from build123d import *

# Parameters (mm, degrees)
BOSS_EXTRUDE1_DEPTH  = 66.675
M6_CLEARANCE_HOLE3_D = 6.6
LPATTERN1_COUNT      = 3
LPATTERN1_PITCH      = 44.45
FILLET1_R            = 2.54


with BuildPart() as part:
    # Sketch1 → Boss-Extrude1 (new, symmetric)
    with BuildSketch(Plane.XY):
        with BuildLine():
            Line((0, 0), (0, 25.4))
            Line((0, 25.4), (3.175, 25.4))
            Line((3.175, 25.4), (3.175, 4.445))
            ThreePointArc((3.175, 4.445), (3.546974388, 3.546974388), (4.445, 3.175))
            Line((4.445, 3.175), (25.4, 3.175))
            Line((25.4, 3.175), (25.4, 0))
            Line((25.4, 0), (0, 0))
        make_face()
    extrude(amount=BOSS_EXTRUDE1_DEPTH, both=True)

    # M6 Clearance Hole3 (through all)
    with Locations(Plane.XZ):
        with Locations((19.05, 60.325), (19.05, 44.45), (19.05, 28.575)):
            m6_clearance_hole3 = Hole(M6_CLEARANCE_HOLE3_D / 2)

    # LPattern1: M6 Clearance Hole3 ×3
    with Locations(*[(0, 0, -i * LPATTERN1_PITCH) for i in range(1, LPATTERN1_COUNT)]):
        add(m6_clearance_hole3, mode=Mode.SUBTRACT)

    # Fillet1
    fillet1_edges = [part.edges().sort_by_distance(p)[0] for p in [
        (1.5875, 25.4, 66.675),
        (1.5875, 25.4, -66.675),
        (25.4, 1.5875, 66.675),
        (25.4, 1.5875, -66.675),
    ]]
    fillet(fillet1_edges, radius=FILLET1_R)


solid = part.part
Part model, mm, in its own coordinate system. A direction names the side the tool comes from. Give positions to 0.01 mm unless a question says otherwise; leave off trailing zeros. Order: outer loops, then holes, each group sorted by start corner. A loop starts at its lowest first (then second) coordinate and runs counter-clockwise, first axis right, second up. Notation, with made-up numbers: (-4, -2) -> (55, -2) arc R26 cw to (55, 34) -> close; hole circle Ø8 at (17, 28). An arc over 180 degrees is marked (long way). Use one line per item in the form item = value.
(1) Saw through at D-D (y = 16.5). Write the cut outline in (x, z) (3 decimals), then the cut area to 3 significant figures.
Solution:
outline = (0, -66.675) -> (3.175, -66.675) -> (3.175, 66.675) -> (0, 66.675) -> close
area = 423 mm²
(2) Saw through at C-C (x = 19.05). Count the separate pieces of the cut face and the enclosed holes in it, then the cut area to 3 significant figures.
Solution:
separate_pieces = 10
enclosed_holes = 0
area = 235 mm²
(3) Flat gauge pins, fed straight in: P1, Ø10.5, axis at y = 18.5, z = -12.5, coming from the +X side (3 decimals); P2, Ø6.5, axis at x = 12.5, z = 13.5, coming from the +Y side (3 decimals); P3, Ø3, axis at x = 5.5, z = 17, coming from the +Y side. Where does each tip first touch, or does it go through?
Solution:
P1 = 3.175
P2 = 3.175
P3 = 3.26
(4) Tool access for faces 4 (the face through (10, 0, 1)), 5 (the face through (3.175, 15, 1)): list every direction of +Z, -Z, +X, -X, +Y, -Y with a clear straight run to the whole face (end or side of a thin tool).
Solution:
face_4 = +Z, -Z, +X, -X, -Y
face_5 = +Z, -Z, +X, +Y
(5) Drill centre lines: line 1 (X direction, y = 23.75, z = 15) (3 decimals); line 2 (Y direction, x = 3.5, z = -30.5). Where is each one in solid material? Low to high. Write a range as from..to.
Solution:
line_1 = 0..3.175
line_2 = 0..3.6
(6) Saw through at B-B (z = 10.5). Write the cut outline in (x, y) (3 decimals), then the cut area to 3 significant figures.
Solution:
outline = (0, 0) -> (25.4, 0) -> (25.4, 3.175) -> (4.445, 3.175) arc R1.27 cw to (3.175, 4.445) -> (3.175, 25.4) -> (0, 25.4) -> close
area = 152 mm²
(7) Pull direction X, two halves, no side cores. Call faces 1 (the face through (3, 7, -66.675)), 2 (the face through (19.765, 1.61, 57.103)), 3 (the face through (24.636, 1.565, -65.951)): +X half, -X half, draft (parallel to the pull), parting line (faces both ways), or undercut.
Solution:
face_1 = draft
face_2 = undercut
face_3 = +X half
(8) Saw through at A-A (z = -44.45). Write the cut outline in (x, y) (3 decimals), then the cut area to 3 significant figures.
Solution:
outline = (0, 0) -> (15.75, 0) -> (15.75, 3.175) -> (4.445, 3.175) arc R1.27 cw to (3.175, 4.445) -> (3.175, 25.4) -> (0, 25.4) -> close; (22.35, 0) -> (25.4, 0) -> (25.4, 3.175) -> (22.35, 3.175) -> close
area = 131 mm²
